Part model, mm, in its own coordinate system. Round coordinates to 2 decimals unless told otherwise and drop trailing zeros. Write each loop counter-clockwise with the first axis right and the second up, starting at its lowest first coordinate (ties: lowest second). Pieces come first, ordered by that corner, then holes.
1) Drill centre lines: L1, parallel to Y at x = -49, z = 2.8; L2, parallel to X at y = 0, z = 1.55; L3, parallel to X at y = 7, z = 1.4. Where is each one in solid material? Low to high.
2) Saw through at C-C on y = -5.5. Write the cut outline in (x, z), and give its area (3 significant figures).
3) Flat gauge pins, fed straight in: pin 1 (3.5 mm diameter, centred on x = -31.5, y = 5, fed in from +Z); pin 2 (3 mm diameter, centred on y = 13.5, z = 0.5, fed in from -X); pin 3 (1 mm diameter, centred on x = 50, z = 3.5, fed in from -Y); pin 4 (1 mm diameter, centred on y = -7, z = 2.5, fed in from +X). Where does each tip first touch, or does it go through?
4) Saw through at A-A on z = 2.95. Count the separate pieces of the cut face and the enclosed holes in it, and give its area (3 significant figures).
5) Saw through at B-B on x = -56. Write the cut outline in (y, z), and give its area (3 significant figures).
6) Saw through at D-D on x = -31.5. Write the cut outline in (y, z), and give its area (3 significant figures).
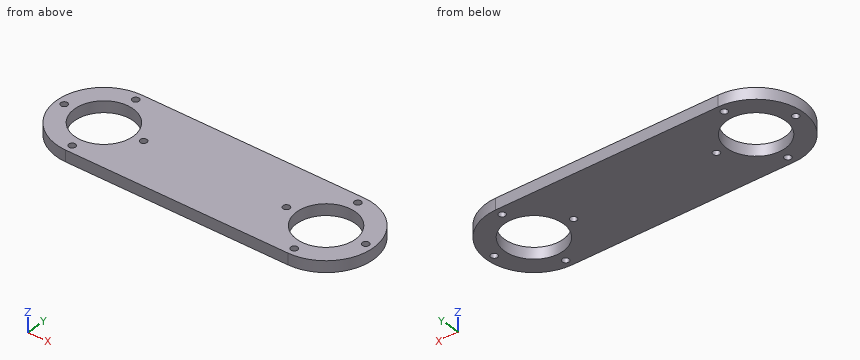
```python
from build123d import *

# Parameters (mm, degrees)
SKETCH1_R           = 1.5
SKETCH1_R_2         = 13
BOSS_EXTRUDE1_DEPTH = 5


with BuildPart() as part:
    # Sketch1 → Boss-Extrude1 (new body)
    with BuildSketch(Plane.XY):
        with BuildLine():
            Line((-49, 26), (49, 26))
            ThreePointArc((49, 26), (70, 5), (49, -16))
            Line((49, -16), (-49, -16))
            ThreePointArc((-49, -16), (-70, 5), (-49, 26))
        make_face()
        with Locations((49, -12.5)):
            Circle(SKETCH1_R, mode=Mode.SUBTRACT)
        with Locations((66.5, 5)):
            Circle(SKETCH1_R, mode=Mode.SUBTRACT)
        with Locations((31.5, 5)):
            Circle(SKETCH1_R, mode=Mode.SUBTRACT)
        with Locations((49, 22.5)):
            Circle(SKETCH1_R, mode=Mode.SUBTRACT)
        with Locations((-49, -12.5)):
            Circle(SKETCH1_R, mode=Mode.SUBTRACT)
        with Locations((-31.5, 5)):
            Circle(SKETCH1_R, mode=Mode.SUBTRACT)
        with Locations((-66.5, 5)):
            Circle(SKETCH1_R, mode=Mode.SUBTRACT)
        with Locations((-49, 22.5)):
            Circle(SKETCH1_R, mode=Mode.SUBTRACT)
        with Locations((-49, 5)):
            Circle(SKETCH1_R_2, mode=Mode.SUBTRACT)
        with Locations((49, 5)):
            Circle(SKETCH1_R_2, mode=Mode.SUBTRACT)
    extrude(amount=BOSS_EXTRUDE1_DEPTH)


solid = part.part
```
Completed:
1. L1: y = -16 to -14, -11 to -8, 18 to 21, 24 to 26
1. L2: x = -69.4 to -61, -37 to 37, 61 to 69.4
1. L3: x = -69.9 to -61.85, -36.15 to 36.15, 61.85 to 69.9
2. outline: (-67.19, 0) - (-56.66, 0) - (-56.66, 5) - (-67.19, 5) - close; (-41.34, 0) - (41.34, 0) - (41.34, 5) - (-41.34, 5) - close; (56.66, 0) - (67.19, 0) - (67.19, 5) - (56.66, 5) - close
2. area: 519 mm2
3. pin 1: stops at z = 5
3. pin 2: stops at x = -68.8
3. pin 3: stops at y = -15.99
3. pin 4: stops at x = 66.57
4. separate pieces: 1
4. enclosed holes: 10
4. area: 4,380 mm2
5. outline: (-14.8, 0) - (-5.95, 0) - (-5.95, 5) - (-14.8, 5) - close; (15.95, 0) - (24.8, 0) - (24.8, 5) - (15.95, 5) - close
5. area: 88.4 mm2
6. outline: (-16, 0) - (3.5, 0) - (3.5, 5) - (-16, 5) - close; (6.5, 0) - (26, 0) - (26, 5) - (6.5, 5) - close
6. area: 195 mm2
